from build123d import *

# Parameters (mm, degrees)
SKETCH1_W           = 52.59
SKETCH1_H           = 52.59
BOSS_EXTRUDE1_DEPTH = 16
SKETCH2_W           = 26
SKETCH2_H           = 6
CUT_EXTRUDE1_DEPTH  = 61.935499711
SKETCH3_R           = 3.5
CUT_EXTRUDE2_DEPTH  = 41.482762381


with BuildPart() as part:
    # Sketch1 → Boss-Extrude1 (new body)
    with BuildSketch(Plane(origin=(0, 0, 0), x_dir=(1, 0, 0), z_dir=(0, 1, 0))):
        Rectangle(SKETCH1_W, SKETCH1_H)
    extrude(amount=BOSS_EXTRUDE1_DEPTH)

    # Sketch2 → Cut-Extrude1 (cut, through all)
    with BuildSketch(Plane(origin=(26.295, 0, 0), x_dir=(0, 0, -1), z_dir=(1, 0, 0))):
        with Locations((0, 13)):
            Rectangle(SKETCH2_W, SKETCH2_H)
    extrude(amount=-CUT_EXTRUDE1_DEPTH, mode=Mode.SUBTRACT)

    # Sketch3 → Cut-Extrude2 (cut, through all)
    with BuildSketch(Plane(origin=(0, 16, 0), x_dir=(1, 0, 0), z_dir=(0, 1, 0))):
        with Locations(Location((-18, 18, 0), (0, 0, 270))):
            Circle(SKETCH3_R)
        with Locations(Location((18, 18, 0), (0, 0, 270))):
            Circle(SKETCH3_R)
        with Locations(Location((18, -18, 0), (0, 0, 270))):
            Circle(SKETCH3_R)
        with Locations(Location((-18, -18, 0), (0, 0, 270))):
            Circle(SKETCH3_R)
    extrude(amount=-CUT_EXTRUDE2_DEPTH, mode=Mode.SUBTRACT)


solid = part.part
CAD build for the part. Positions are in the model's coordinates, mm. A direction names the side the tool comes from. Round coordinates to 2 decimals unless told otherwise and drop trailing zeros. Loops run counter-clockwise (first coordinate to the right, second up) from the corner with the lowest first, then second, coordinate; pieces in that order, holes last. Notation, with made-up numbers: M -1.5,-7.5 L 8.5,-7.5 A22 ccw 8.5,18.5 Z; hole C 59.5,59 d2. An arc over 180 degrees is marked long. One line per question, with ' | ' between items. Start each with the question number.
Item 1: Cut at D-D, the plane x = -18. Write the cut outline in (y, z) (3 decimals), plus the area to 3 significant figures.
Item 2: Two-plate mould, pull along Z, no slides. Class faces 3 (the flat face through (0, 8, 26.295)), 4 (the cylindrical face through (20.95, 8.11, 19.88)), 5 (the flat face through (0, 0, 0)): pulls with the +Z half, pulls with the -Z half, needs draft (parallel to the pull), parting line crosses it, or undercut.
Item 3: Which spindle directions (+Z, -Z, +X, -X, +Y, -Y) get a long thin tool onto all of the face, cutting with end or side? Do faces 1 (the flat face through (0, 13, 13)), 2 (the cylindrical face through (-15.05, 8.11, -16.12)). Say none if no direction does.
Item 4: Cut at B-B, the plane z = 18. Write the cut outline in (x, y) (3 decimals), plus the area to 3 significant figures.
Item 5: Pin check, flat tip, straight feed: pin 1 Ø13 at (x, z) = (-11.5, -2.5) entering from +Y. Stop position of the tip, or through.
Item 6: Wall check: line 1 (X direction, y = 6.5, z = 18) (3 decimals); line 2 (X direction, y = 4.5, z = -19.5) (3 decimals); line 3 (Z direction, x = -8.5, y = 14.5) (3 decimals). Give the ranges that are in metal, low to high.
Item 7: Cut at C-C, the plane y = 5.25. Write the cut outline in (x, z) (3 decimals), plus the area to 3 significant figures.
Item 8: Cut at A-A, the plane y = 11.5. Write the cut outline in (x, z) (3 decimals), plus the area to 3 significant figures.
Responses:
1) outline: M 0,-26.295 L 16,-26.295 L 16,-21.5 L 0,-21.5 Z; M 0,-14.5 L 16,-14.5 L 16,-13 L 10,-13 L 10,13 L 16,13 L 16,14.5 L 0,14.5 Z; M 0,21.5 L 16,21.5 L 16,26.295 L 0,26.295 Z | area: 461 mm²
2) face 3: pulls with the +Z half | face 4: undercut | face 5: needs draft
3) face 1: +X, -X, +Y | face 2: +Y, -Y
4) outline: M -26.295,0 L -21.5,0 L -21.5,16 L -26.295,16 Z; M -14.5,0 L 14.5,0 L 14.5,16 L -14.5,16 Z; M 21.5,0 L 26.295,0 L 26.295,16 L 21.5,16 Z | area: 617 mm²
5) pin 1: stops at y = 10
6) line 1: x = -26.295 to -21.5, -14.5 to 14.5, 21.5 to 26.295 | line 2: x = -26.295 to -21.162, -14.838 to 14.838, 21.162 to 26.295 | line 3: z = -26.295 to -13, 13 to 26.295
7) outline: M -26.295,-26.295 L 26.295,-26.295 L 26.295,26.295 L -26.295,26.295 Z; hole C -18,-18 d7; hole C -18,18 d7; hole C 18,-18 d7; hole C 18,18 d7 | area: 2,610 mm²
8) outline: M -26.295,-26.295 L 26.295,-26.295 L 26.295,-13 L -26.295,-13 Z; M -26.295,13 L 26.295,13 L 26.295,26.295 L -26.295,26.295 Z; hole C -18,-18 d7; hole C -18,18 d7; hole C 18,-18 d7; hole C 18,18 d7 | area: 1,240 mm²
